```python
from build123d import *

# Parameters (mm, degrees)
BOSS_EXTRUDE1_DEPTH = 5
SKETCH2_R           = 10.5
CUT_EXTRUDE1_DEPTH  = 2.5
SKETCH3_R           = 2.25
SKETCH3_R_2         = 1.25
CUT_EXTRUDE2_DEPTH  = 59.792006259
SKETCH7_W           = 35
SKETCH7_H           = 3
CUT_EXTRUDE4_DEPTH  = 59.951251047
SKETCH6_W           = 7.5
SKETCH6_H           = 3
CUT_EXTRUDE3_DEPTH  = 59.951251047
SKETCH8_R           = 1.75
CUT_EXTRUDE5_DEPTH  = 59.951251047
FILLET3_R           = 3
CHAMFER1_SIZE       = 3


with BuildPart() as part:
    # Sketch1 → Boss-Extrude1 (new body)
    with BuildSketch(Plane(origin=(0, 0, 0), x_dir=(1, 0, 0), z_dir=(0, 1, 0))):
        Polygon((0, 12), (57.5, 12), (57.5, -12), (0, -12), (-49, -12), (-49, 12), align=None)
    extrude(amount=BOSS_EXTRUDE1_DEPTH)

    # Sketch2 → Cut-Extrude1 (cut)
    with BuildSketch(Plane.XZ):
        with Locations(Location((45.5, 0, 0), (0, 0, 270))):
            Circle(SKETCH2_R)
        with Locations(Location((-37, 0, 0), (0, 0, 90))):
            Circle(SKETCH2_R)
    extrude(amount=-CUT_EXTRUDE1_DEPTH, mode=Mode.SUBTRACT)

    # Sketch3 → Cut-Extrude2 (cut, through all)
    with BuildSketch(Plane.XZ.offset(-2.5)):
        with Locations(Location((45.5, 0, 0), (0, 0, 270))):
            Circle(SKETCH3_R)
        with Locations(Location((45.5, 7.25, 0), (0, 0, 270))):
            Circle(SKETCH3_R_2)
        with Locations(Location((42, 7.25, 0), (0, 0, 270))):
            Circle(SKETCH3_R_2)
        with Locations(Location((49, 7.25, 0), (0, 0, 270))):
            Circle(SKETCH3_R_2)
        with Locations(Location((52.75, 0, 0), (0, 0, 270))):
            Circle(SKETCH3_R_2)
        with Locations(Location((52.75, -3.5, 0), (0, 0, 270))):
            Circle(SKETCH3_R_2)
        with Locations(Location((52.75, 3.5, 0), (0, 0, 270))):
            Circle(SKETCH3_R_2)
        with Locations(Location((45.5, -7.25, 0), (0, 0, 270))):
            Circle(SKETCH3_R_2)
        with Locations(Location((42, -7.25, 0), (0, 0, 270))):
            Circle(SKETCH3_R_2)
        with Locations(Location((49, -7.25, 0), (0, 0, 270))):
            Circle(SKETCH3_R_2)
        with Locations(Location((38.25, 0, 0), (0, 0, 270))):
            Circle(SKETCH3_R_2)
        with Locations(Location((38.25, 3.5, 0), (0, 0, 270))):
            Circle(SKETCH3_R_2)
        with Locations(Location((38.25, -3.5, 0), (0, 0, 270))):
            Circle(SKETCH3_R_2)
        with Locations(Location((-37, 0, 0), (0, 0, 270))):
            Circle(SKETCH3_R)
        with Locations(Location((-37, 7.25, 0), (0, 0, 270))):
            Circle(SKETCH3_R_2)
        with Locations(Location((-40.5, 7.25, 0), (0, 0, 270))):
            Circle(SKETCH3_R_2)
        with Locations(Location((-33.5, 7.25, 0), (0, 0, 270))):
            Circle(SKETCH3_R_2)
        with Locations(Location((-29.75, 3.5, 0), (0, 0, 270))):
            Circle(SKETCH3_R_2)
        with Locations(Location((-29.75, 0, 0), (0, 0, 270))):
            Circle(SKETCH3_R_2)
        with Locations(Location((-29.75, -3.5, 0), (0, 0, 270))):
            Circle(SKETCH3_R_2)
        with Locations(Location((-33.5, -7.25, 0), (0, 0, 270))):
            Circle(SKETCH3_R_2)
        with Locations(Location((-37, -7.25, 0), (0, 0, 270))):
            Circle(SKETCH3_R_2)
        with Locations(Location((-40.5, -7.25, 0), (0, 0, 270))):
            Circle(SKETCH3_R_2)
        with Locations(Location((-44.25, -3.5, 0), (0, 0, 270))):
            Circle(SKETCH3_R_2)
        with Locations(Location((-44.25, 0, 0), (0, 0, 270))):
            Circle(SKETCH3_R_2)
        with Locations(Location((-44.25, 3.5, 0), (0, 0, 270))):
            Circle(SKETCH3_R_2)
    extrude(amount=-CUT_EXTRUDE2_DEPTH, mode=Mode.SUBTRACT)

    # Sketch7 → Cut-Extrude4 (cut, through all)
    with BuildSketch(Plane.XZ):
        with Locations((0, 10.5)):
            Rectangle(SKETCH7_W, SKETCH7_H)
        with Locations((0, -10.5)):
            Rectangle(SKETCH7_W, SKETCH7_H)
    extrude(amount=-CUT_EXTRUDE4_DEPTH, mode=Mode.SUBTRACT)

    # Sketch6 → Cut-Extrude3 (cut, through all)
    with BuildSketch(Plane.XZ):
        with Locations((0, 7.5)):
            Rectangle(SKETCH6_W, SKETCH6_H)
        with Locations((0, -7.5)):
            Rectangle(SKETCH6_W, SKETCH6_H)
    extrude(amount=-CUT_EXTRUDE3_DEPTH, mode=Mode.SUBTRACT)

    # Sketch8 → Cut-Extrude5 (cut, through all)
    with BuildSketch(Plane(origin=(0, 5, 0), x_dir=(1, 0, 0), z_dir=(0, 1, 0))):
        with Locations(Location((11.25, 0, 0), (0, 0, 270))):
            Circle(SKETCH8_R)
        with Locations(Location((-11.25, 0, 0), (0, 0, 90))):
            Circle(SKETCH8_R)
    extrude(amount=-CUT_EXTRUDE5_DEPTH, mode=Mode.SUBTRACT)

    # Fillet3
    fillet3_edges = [part.edges().sort_by_distance(p)[0] for p in [
        (-49, 2.5, 12),
        (-49, 2.5, -12),
        (57.5, 2.5, -12),
        (57.5, 2.5, 12),
    ]]
    fillet(fillet3_edges, radius=FILLET3_R)

    # Chamfer1
    chamfer1_edges = [part.edges().sort_by_distance(p)[0] for p in [
        (-17.5, 2.5, 12),
        (17.5, 2.5, 12),
        (17.5, 2.5, -12),
        (-17.5, 2.5, -12),
    ]]
    chamfer(chamfer1_edges, length=CHAMFER1_SIZE - 0.0001)  # a hair under: the kernel refuses the full size


solid = part.part
```
Geometry check sheet. Reference: the model listing, model coordinates, mm. A direction names the side the tool comes from. Round coordinates to 2 decimals unless told otherwise and drop trailing zeros. Order: outer loops, then holes, each group sorted by start corner. A loop starts at its lowest first (then second) coordinate and runs counter-clockwise, first axis right, second up. Notation, with made-up numbers: (0, 12) - (41, 12) arc R17 ccw to (41, 45) - close; hole circle Ø10 at (-34.75, 32). An arc over 180 degrees is marked (long way). Use a Markdown table: item, result. Add a question column.
(1) Material ranges on line 1 along X through (y, z) = (4.45, -3.5); line 2 along Z through (x, y) = (-41.5, 0.5); line 3 along X through (y, z) = (1.65, 0), recorded low to high. Write a range as [from, to].
(2) Depth check by flat-ended pin: pin 1 (3 mm diameter, centred on x = 52.75, z = 0, fed in from +Y); pin 2 (3 mm diameter, centred on x = -40.5, z = 7.25, fed in from -Y). Enter the tip coordinate at first touch or a pass-through.
(3) Sectioned sample at A-A, the plane y = 1.35. Count the separate pieces of the cut face and the enclosed holes in it, and give its area (3 significant figures).
(4) Release check for a two-part mould opening along Z. For faces 4 (the flat face through (11, 2, 9)), 5 (the flat face through (-3.75, 2, 7)), 6 (the cylindrical face through (54, 4, 0)), 7 (the flat face through (11, 2, -9)) record: pulls with the +Z half, pulls with the -Z half, needs draft (parallel to the pull), parting line crosses it, or undercut.
(5) Sectioned sample at B-B, the plane x = 52.75. Enter the section's corners in (y, z), and give its area (3 significant figures).
(6) Sectioned sample at C-C, the plane x = -33.5. Enter the section's corners in (y, z), and give its area (3 significant figures).
(7) Tool access check on faces 1 (the cylindrical face through (53.99, 3.73, 3.66)), 2 (the cylindrical face through (36.185, 1.232, -4.845)), 3 (the flat face through (-19, 2.5, 10.5)). Record the directions out of +Z, -Z, +X, -X, +Y, -Y that give a thin tool (end or side, any length) a straight path to the whole face; none if there is none.
(8) Sectioned sample at D-D, the plane z = -3.5. Enter the section's corners in (x, y).
Answers below:
| question | item | result |
|---|---|---|
| 1 | line 1 | [-49, -45.5], [-43, -31], [-28.5, 37], [39.5, 51.5], [54, 57.5] |
| 1 | line 2 | [-12, -9.49], [9.49, 12] |
| 1 | line 3 | [-49, -47.5], [-26.5, -13], [-9.5, 9.5], [13, 35], [56, 57.5] |
| 2 | pin 1 | y = 5 |
| 2 | pin 2 | y = 2.5 |
| 3 | separate pieces | 1 |
| 3 | enclosed holes | 4 |
| 3 | area | 1,560 mm² |
| 4 | face 4 | pulls with the +Z half |
| 4 | face 5 | needs draft |
| 4 | face 6 | undercut |
| 4 | face 7 | pulls with the -Z half |
| 5 | outline | (0, -12) - (5, -12) - (5, -4.75) - (2.5, -4.75) - (2.5, -7.6) - (0, -7.6) - close; (0, 7.6) - (2.5, 7.6) - (2.5, 4.75) - (5, 4.75) - (5, 12) - (0, 12) - close; (2.5, -2.25) - (5, -2.25) - (5, -1.25) - (2.5, -1.25) - close; (2.5, 1.25) - (5, 1.25) - (5, 2.25) - (2.5, 2.25) - close |
| 5 | area | 63.3 mm² |
| 6 | outline | (0, -12) - (5, -12) - (5, -8.5) - (2.5, -8.5) - (2.5, -9.9) - (0, -9.9) - close; (0, 9.9) - (2.5, 9.9) - (2.5, 8.5) - (5, 8.5) - (5, 12) - (0, 12) - close; (2.5, -6) - (5, -6) - (5, 6) - (2.5, 6) - close |
| 6 | area | 58.0 mm² |
| 7 | face 1 | +Y, -Y |
| 7 | face 2 | -Y |
| 7 | face 3 | +Z, +Y, -Y |
| 8 | outline | (-49, 0) - (-46.9, 0) - (-46.9, 2.5) - (-45.5, 2.5) - (-45.5, 5) - (-49, 5) - close; (-43, 2.5) - (-31, 2.5) - (-31, 5) - (-43, 5) - close; (-28.5, 2.5) - (-27.1, 2.5) - (-27.1, 0) - (35.6, 0) - (35.6, 2.5) - (37, 2.5) - (37, 5) - (-28.5, 5) - close; (39.5, 2.5) - (51.5, 2.5) - (51.5, 5) - (39.5, 5) - close; (54, 2.5) - (55.4, 2.5) - (55.4, 0) - (57.5, 0) - (57.5, 5) - (54, 5) - close |
